Part model, mm, in its own coordinate system. A direction names the side the tool comes from. Give positions to 0.01 mm unless a question says otherwise; leave off trailing zeros. Write each loop counter-clockwise with the first axis right and the second up, starting at its lowest first coordinate (ties: lowest second). Pieces come first, ordered by that corner, then holes. Notation, with made-up numbers: (-8, 4) - (50, 4) arc R31 ccw to (50, 41) - close; hole circle Ø3 at (-20, 43.5). An arc over 180 degrees is marked (long way). Answer as a JSON object with one key per item and string values. Group by question number.
```python
from build123d import *

# Parameters (mm, degrees)
F0_W     = 55.9842921793
F0_H     = 102.7474403381
F1_DEPTH = 12.7
F2_R     = 5.08
F3_W     = 45.8242921793
F3_H     = 14.4344866276
F4_DEPTH = 25.4
F8_DEPTH = 56.8421371281


with BuildPart() as f1:
    # F0 (on Front) → F1 (new body)
    with BuildSketch(Plane.XZ):
        Rectangle(F0_W, F0_H)
    extrude(amount=F1_DEPTH)

    # F2
    f2_edges = [f1.edges().sort_by_distance(p)[0] for p in [
        (27.992146, -12.7, 0),
        (27.992146, 0, 0),
        (-27.992146, -12.7, 0),
        (-27.992146, 0, 0),
    ]]
    fillet(f2_edges, radius=F2_R)

    # F3 (on face) → F4 (cut)
    with BuildSketch(Plane.XZ.offset(12.7)):
        with Locations((0, -44.1564768553)):
            Rectangle(F3_W, F3_H)
    extrude(amount=-F4_DEPTH, mode=Mode.SUBTRACT)

    # F8 (add): a face of the model
    f8_faces = [f1.faces().sort_by_distance(p)[0] for p in [
        (0, -6.35, 51.3737201691),
    ]]
    extrude(f8_faces, amount=F8_DEPTH)


solid = f1.part
```
1) Probe line 1 (Z direction, x = 5, y = -11.5); line 2 (Y direction, x = 23, z = 6); line 3 (X direction, y = -7.75, z = 99). List the from-to ranges inside material, lowest first.
2) Band-saw the part on A-A (z = 93). List the corners of the cut face in (x, y).
3) Drop a flat-ended pin along its axis: P1, Ø4, axis at x = 8, y = -6.5, coming from the -Z side. Give the stop position or say it passes through.
4) Band-saw the part on B-B (y = -3.5). List the corners of the cut face in (x, z), plus the area to 3 significant figures.
5) Which spindle directions (+Z, -Z, +X, -X, +Y, -Y) get a long thin tool onto all of the face, cutting with end or side? Do faces 1 (the flat face through (0, -6, -36.939)), 2 (the flat face through (0, 0, 37)). Say none if no direction does.
6) Mould opens along X. For faces 3 (the cylindrical face through (-26.544, -1.528, 27.304)), 4 (the flat face through (-22.912, -6, -44)), 5 (the flat face through (0, -6, 108.216)) say: pulls with the +X half, pulls with the -X half, needs draft (parallel to the pull), parting line crosses it, or undercut.
7) Band-saw the part on C-C (x = -4). List the corners of the cut face in (y, z), plus the area to 3 significant figures.
Verdict:
{
 "1": {"line 1": "-36.94 to 108.22", "line 2": "-12.7 to 0", "line 3": "-27.99 to 27.99"},
 "2": {"outline": "(-27.99, -7.62) arc R5.08 ccw to (-22.91, -12.7) - (22.91, -12.7) arc R5.08 ccw to (27.99, -7.62) - (27.99, -5.08) arc R5.08 ccw to (22.91, 0) - (-22.91, 0) arc R5.08 ccw to (-27.99, -5.08) - close"},
 "3": {"P1": "z = -36.94"},
 "4": {"outline": "(-27.74, -51.37) - (-22.91, -51.37) - (-22.91, -36.94) - (22.91, -36.94) - (22.91, -51.37) - (27.74, -51.37) - (27.74, 108.22) - (-27.74, 108.22) - close", "area": "8,190 mm2"},
 "5": {"face 1": "-Z, +Y, -Y", "face 2": "+Z, -Z, +X, -X, +Y"},
 "6": {"face 3": "pulls with the -X half", "face 4": "undercut", "face 5": "needs draft"},
 "7": {"outline": "(-12.7, -36.94) - (0, -36.94) - (0, 108.22) - (-12.7, 108.22) - close", "area": "1,840 mm2"}
}
